Verification items for the finished model (mm, model axes). A direction names the side the tool comes from. Give positions to 0.01 mm unless a question says otherwise; leave off trailing zeros. Loops run counter-clockwise (first coordinate to the right, second up) from the corner with the lowest first, then second, coordinate; pieces in that order, holes last. Notation, with made-up numbers: (-18.5, 55) -> (33.5, 55) arc R21 cw to (33.5, 68) -> close; hole circle Ø7 at (45.25, -1.75). An arc over 180 degrees is marked (long way). Answer in a Markdown table with one row per item. Add a question column.
Q1. Section check C-C on y = 27.5. Enter the section's corners in (x, z).
Q2. Release check for a two-part mould opening along X. For faces 4 (the face through (-1, 0, 54)), 5 (the face through (38.59, 3.7, 101.94)), 6 (the face through (42.73, 3.7, 8.79)), 7 (the face through (27.5, 30, 54)) record: pulls with the +X half, pulls with the -X half, needs draft (parallel to the pull), parting line crosses it, or undercut.
Q3. Set-up check for faces 1 (the face through (-27.5, 30, 54)), 2 (the face through (40, 7.5, 54)), 3 (the face through (-52.5, 4, 54)): record each of +Z, -Z, +X, -X, +Y, -Y from which the full face is reachable in a straight line by a thin tool's end or side.
Q4. Section check D-D on z = 30. Enter the section's corners in (x, y), and give its area (3 significant figures).
Q5. Section check B-B on z = 15. Enter the section's corners in (x, y), and give its area (3 significant figures).
Q6. Section check A-A on x = 39.5. Enter the section's corners in (y, z), and give its area (3 significant figures).
Q7. Material ranges on probe 1 along Z at (x, y) = (39.5, 2.5); probe 2 along Y at (x, z) = (0, 32); probe 3 along Z at (x, y) = (45.5, 3), recorded low to high.
Q8. Gauge pin test, flat ends, axial feed: P1, Ø20, axis at x = 44, z = 79, coming from the +Y side; P2, Ø22.5, axis at y = 30.5, z = 59, coming from the -X side. Record the tip position at first contact, or that the pin passes through.
```python
from build123d import *

# Parameters (mm, degrees)
F0_R     = 17.5
F1_DEPTH = 110
F2_R     = 7
F3_DEPTH = 25


with BuildPart() as f1:
    # F0 (on Top) → F1 (new body)
    with BuildSketch(Plane.XY):
        Polygon((-52.5, 7.5), (-52.5, 0), (0, 0), (52.5, 0), (52.5, 7.5), (27.5, 7.5), (27.5, 52.5), (0, 52.5), (-27.5, 52.5), (-27.5, 7.5), align=None)
        with Locations((0, 27.5)):
            Circle(F0_R, mode=Mode.SUBTRACT)
    extrude(amount=F1_DEPTH)

    # F2 (on face) → F3 (cut)
    with BuildSketch(Plane.XZ):
        with Locations((-40.5, 95)):
            Circle(F2_R)
        with Locations((39.5, 95)):
            Circle(F2_R)
        with Locations((-40.5, 15)):
            Circle(F2_R)
        with Locations((39.5, 15)):
            Circle(F2_R)
    extrude(amount=-F3_DEPTH, mode=Mode.SUBTRACT)


solid = f1.part
```
Taken from the geometry:
| question | item | result |
|---|---|---|
| 1 | outline | (-27.5, 0) -> (-17.5, 0) -> (-17.5, 110) -> (-27.5, 110) -> close; (17.5, 0) -> (27.5, 0) -> (27.5, 110) -> (17.5, 110) -> close |
| 2 | face 4 | needs draft |
| 2 | face 5 | undercut |
| 2 | face 6 | undercut |
| 2 | face 7 | pulls with the +X half |
| 3 | face 1 | +Z, -Z, -X, +Y |
| 3 | face 2 | +Z, -Z, +X, +Y |
| 3 | face 3 | +Z, -Z, -X, +Y, -Y |
| 4 | outline | (-52.5, 0) -> (52.5, 0) -> (52.5, 7.5) -> (27.5, 7.5) -> (27.5, 52.5) -> (-27.5, 52.5) -> (-27.5, 7.5) -> (-52.5, 7.5) -> close; hole circle Ø35 at (0, 27.5) |
| 4 | area | 2,300 mm² |
| 5 | outline | (-52.5, 0) -> (-47.5, 0) -> (-47.5, 7.5) -> (-52.5, 7.5) -> close; (-33.5, 0) -> (32.5, 0) -> (32.5, 7.5) -> (27.5, 7.5) -> (27.5, 52.5) -> (-27.5, 52.5) -> (-27.5, 7.5) -> (-33.5, 7.5) -> close; (46.5, 0) -> (52.5, 0) -> (52.5, 7.5) -> (46.5, 7.5) -> close; hole circle Ø35 at (0, 27.5) |
| 5 | area | 2,090 mm² |
| 6 | outline | (0, 0) -> (7.5, 0) -> (7.5, 8) -> (0, 8) -> close; (0, 22) -> (7.5, 22) -> (7.5, 88) -> (0, 88) -> close; (0, 102) -> (7.5, 102) -> (7.5, 110) -> (0, 110) -> close |
| 6 | area | 615 mm² |
| 7 | probe 1 | z = 0 to 8, 22 to 88, 102 to 110 |
| 7 | probe 2 | y = 0 to 10, 45 to 52.5 |
| 7 | probe 3 | z = 0 to 11.39, 18.61 to 91.39, 98.61 to 110 |
| 8 | P1 | stops at y = 7.5 |
| 8 | P2 | stops at x = -27.5 |
